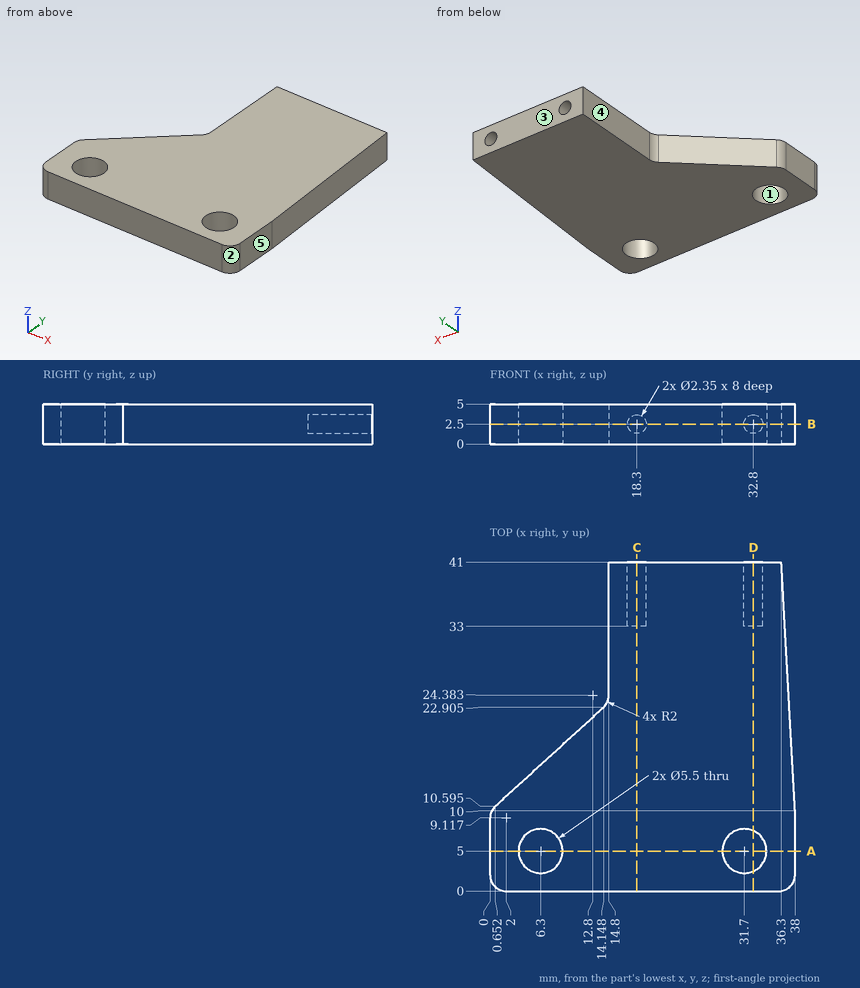
Job drawing, mm, ordinate dimensions from the low corner. One solid piece. A direction names the side the tool comes from. Coordinates: 2 decimals unless noted, no trailing zeros. Order: outer loops, then holes, each group sorted by start corner. A loop starts at its lowest first (then second) coordinate and runs counter-clockwise, first axis right, second up. Notation, with made-up numbers: M 71.25,-9 L 108.25,-9 A17 ccw 108.25,2 Z; hole C -25,40.5 d3. An arc over 180 degrees is marked long. Return JSON: item names as keys, results as strings.
1. Pull direction X, two halves, no side cores. Call the marked faces 1, 2 and 3: +X half, -X half, draft (parallel to the pull), parting line (faces both ways), or undercut.
Ans:
{"face 1": "undercut", "face 2": "+X half", "face 3": "draft"}
2. Saw through at D-D (x = 32.8). Give the cut face in (y, z) (1 decimal), and give its area (3 significant figures).
Ans:
{"outline": "M 0,0 L 2.5,0 L 2.5,5 L 0,5 Z; M 7.5,0 L 41,0 L 41,1.3 L 33,1.3 L 33,3.7 L 41,3.7 L 41,5 L 7.5,5 Z", "area": "161 mm^2"}
3. Saw through at C-C (x = 18.3). Give the cut face in (y, z) (1 decimal).
Ans:
{"outline": "M 0,0 L 41,0 L 41,1.3 L 33,1.3 L 33,3.7 L 41,3.7 L 41,5 L 0,5 Z"}
4. Drill centre lines: probe 1 along Y at (x, z) = (31.7, 3.6); probe 2 along X at (y, z) = (35.75, 2.5) (1 decimal); probe 3 along X at (y, z) = (7, 0.4). Where is each one in solid material? Low to high.
Ans:
{"probe 1": "0 to 2.25, 7.75 to 41", "probe 2": "14.8 to 17.1, 19.5 to 31.6, 34 to 36.6", "probe 3": "0 to 4.41, 8.19 to 29.81, 33.59 to 38"}
5. Flat gauge pins, fed straight in: pin 1 (1.9 mm diameter, centred on x = 32.8, z = 2.5, fed in from +Y); pin 2 (2 mm diameter, centred on y = 24, z = 1, fed in from -X) (1 decimal); pin 3 (1.5 mm diameter, centred on y = 33.5, z = 3.5, fed in from +X); pin 4 (5 mm diameter, centred on x = 31.7, y = 5, fed in from -Z). Where does each tip first touch, or does it go through?
Ans:
{"pin 1": "y = 33", "pin 2": "x = 14.2", "pin 3": "x = 36.75", "pin 4": "through"}
6. Saw through at A-A (y = 5). Give the cut face in (x, z), and give its area (3 significant figures).
Ans:
{"outline": "M 0,0 L 3.55,0 L 3.55,5 L 0,5 Z; M 9.05,0 L 28.95,0 L 28.95,5 L 9.05,5 Z; M 34.45,0 L 38,0 L 38,5 L 34.45,5 Z", "area": "135 mm^2"}
7. Tool access for the marked faces 4 and 5: list every direction of +Z, -Z, +X, -X, +Y, -Y with a clear straight run to the whole face (end or side of a thin tool).
Ans:
{"face 4": "+Z, -Z, -X, +Y", "face 5": "+Z, -Z, +X, +Y, -Y"}
8. Saw through at B-B (z = 2.5). Give the number of separate pieces and of enclosed holes in the cut face, and give its area (3 significant figures).
Ans:
{"separate pieces": "1", "enclosed holes": "2", "area": "1,090 mm^2"}
